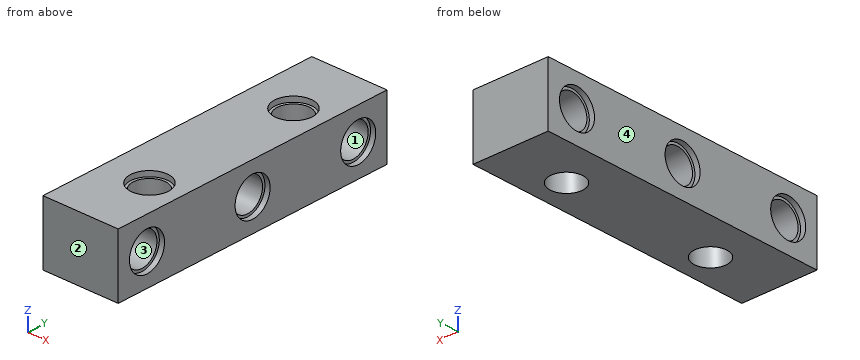
from build123d import *

# Parameters (mm, degrees)
ESQUISSE1_W                  = 12
ESQUISSE1_H                  = 40
BOSS_EXTRU_1_DEPTH           = 12
ESQUISSE3_R                  = 3.15
ENL_V_MAT_EXTRU_1_DEPTH      = 44.451121965
ENL_V_MAT_EXTRU_1_DEPTH_BACK = 44.451121965
ESQUISSE4_R                  = 3.15
ENL_V_MAT_EXTRU_2_DEPTH      = 44.451121965
ENL_V_MAT_EXTRU_2_DEPTH_BACK = 44.451121965
ESQUISSE5_R                  = 3.65
ENL_V_MAT_EXTRU_3_DEPTH      = 1
ESQUISSE6_R                  = 3.65
ENL_V_MAT_EXTRU_4_DEPTH      = 1
ESQUISSE7_W                  = 12
ESQUISSE7_H                  = 8
BOSS_EXTRU_2_DEPTH           = 12
ESQUISSE8_W                  = 1
ESQUISSE8_H                  = 12
ENL_V_MAT_EXTRU_5_DEPTH      = 59.514955353
ENL_V_MAT_EXTRU_5_DEPTH_BACK = 59.514955353
ESQUISSE9_R                  = 3.15
ENL_V_MAT_EXTRU_6_DEPTH      = 51.68530359
ENL_V_MAT_EXTRU_6_DEPTH_BACK = 51.68530359
ESQUISSE11_W                 = 12
ESQUISSE11_H                 = 56
ESQUISSE11_R                 = 3.15
BOSS_EXTRU_3_DEPTH           = 3.5
ESQUISSE12_R                 = 3.65
ENL_V_MAT_EXTRU_8_DEPTH      = 1
ESQUISSE13_R                 = 3.65
ENL_V_MAT_EXTRU_9_DEPTH      = 1


with BuildPart() as part:
    # Esquisse1 → Boss.-Extru.1 (new body)
    with BuildSketch(Plane.XY):
        with Locations((6, 20)):
            Rectangle(ESQUISSE1_W, ESQUISSE1_H)
    extrude(amount=BOSS_EXTRU_1_DEPTH)

    # Esquisse3 → Enlèv. mat.-Extru.1 (cut, two sides)
    with BuildSketch(Plane.XY.offset(12)) as enl_v_mat_extru_1_sk:
        with Locations((5, 5)):
            Circle(ESQUISSE3_R)
        with Locations((5, 35)):
            Circle(ESQUISSE3_R)
    extrude(amount=ENL_V_MAT_EXTRU_1_DEPTH, mode=Mode.SUBTRACT)
    extrude(enl_v_mat_extru_1_sk.sketch, amount=-ENL_V_MAT_EXTRU_1_DEPTH_BACK, mode=Mode.SUBTRACT)

    # Esquisse4 → Enlèv. mat.-Extru.2 (cut, two sides)
    with BuildSketch(Plane(origin=(12, 0, 0), x_dir=(0, 0, -1), z_dir=(1, 0, 0))) as enl_v_mat_extru_2_sk:
        with Locations((-6, 20)):
            Circle(ESQUISSE4_R)
    extrude(amount=ENL_V_MAT_EXTRU_2_DEPTH, mode=Mode.SUBTRACT)
    extrude(enl_v_mat_extru_2_sk.sketch, amount=-ENL_V_MAT_EXTRU_2_DEPTH_BACK, mode=Mode.SUBTRACT)

    # Esquisse5 → Enlèv. mat.-Extru.3 (cut)
    with BuildSketch(Plane.XY.offset(12)):
        with Locations((5, 35)):
            Circle(ESQUISSE5_R)
        with Locations((5, 5)):
            Circle(ESQUISSE5_R)
    extrude(amount=-ENL_V_MAT_EXTRU_3_DEPTH, mode=Mode.SUBTRACT)

    # Esquisse6 → Enlèv. mat.-Extru.4 (cut)
    with BuildSketch(Plane(origin=(12, 0, 0), x_dir=(0, 0, -1), z_dir=(1, 0, 0))):
        with Locations((-6, 20)):
            Circle(ESQUISSE6_R)
    extrude(amount=-ENL_V_MAT_EXTRU_4_DEPTH, mode=Mode.SUBTRACT)

    # Esquisse7 → Boss.-Extru.2 (add)
    with BuildSketch(Plane(origin=(12, 0, 0), x_dir=(0, 0, -1), z_dir=(1, 0, 0))):
        with Locations((-6, -4)):
            Rectangle(ESQUISSE7_W, ESQUISSE7_H)
        with Locations((-6, 44)):
            Rectangle(ESQUISSE7_W, ESQUISSE7_H)
    extrude(amount=-BOSS_EXTRU_2_DEPTH)

    # Esquisse8 → Enlèv. mat.-Extru.5 (cut, two sides)
    with BuildSketch(Plane.XZ.offset(8)) as enl_v_mat_extru_5_sk:
        with Locations((11.5, 6)):
            Rectangle(ESQUISSE8_W, ESQUISSE8_H)
    extrude(amount=ENL_V_MAT_EXTRU_5_DEPTH, mode=Mode.SUBTRACT)
    extrude(enl_v_mat_extru_5_sk.sketch, amount=-ENL_V_MAT_EXTRU_5_DEPTH_BACK, mode=Mode.SUBTRACT)

    # Esquisse9 → Enlèv. mat.-Extru.6 (cut, two sides)
    with BuildSketch(Plane(origin=(11, 0, 0), x_dir=(0, 0, -1), z_dir=(1, 0, 0))) as enl_v_mat_extru_6_sk:
        with Locations((-6, 42)):
            Circle(ESQUISSE9_R)
        with Locations((-6, -2)):
            Circle(ESQUISSE9_R)
    extrude(amount=ENL_V_MAT_EXTRU_6_DEPTH, mode=Mode.SUBTRACT)
    extrude(enl_v_mat_extru_6_sk.sketch, amount=-ENL_V_MAT_EXTRU_6_DEPTH_BACK, mode=Mode.SUBTRACT)

    # Esquisse11 → Boss.-Extru.3 (add)
    with BuildSketch(Plane.ZY):
        with Locations((6, 20)):
            Rectangle(ESQUISSE11_W, ESQUISSE11_H)
        with Locations(Location((6, -2, 0), (0, 0, 180))):
            Circle(ESQUISSE11_R, mode=Mode.SUBTRACT)
        with Locations(Location((6, 20, 0), (0, 0, 180))):
            Circle(ESQUISSE11_R, mode=Mode.SUBTRACT)
        with Locations(Location((6, 42, 0), (0, 0, 180))):
            Circle(ESQUISSE11_R, mode=Mode.SUBTRACT)
    extrude(amount=BOSS_EXTRU_3_DEPTH)

    # Esquisse12 → Enlèv. mat.-Extru.8 (cut)
    with BuildSketch(Plane.ZY.offset(3.5)):
        with Locations((6, 42)):
            Circle(ESQUISSE12_R)
        with Locations((6, 20)):
            Circle(ESQUISSE12_R)
        with Locations((6, -2)):
            Circle(ESQUISSE12_R)
    extrude(amount=-ENL_V_MAT_EXTRU_8_DEPTH, mode=Mode.SUBTRACT)

    # Esquisse13 → Enlèv. mat.-Extru.9 (cut)
    with BuildSketch(Plane(origin=(11, 0, 0), x_dir=(0, 0, -1), z_dir=(1, 0, 0))):
        with Locations(Location((-6, -2, 0), (0, 0, 180))):
            Circle(ESQUISSE13_R)
        with Locations(Location((-6, 20, 0), (0, 0, 180))):
            Circle(ESQUISSE13_R)
        with Locations(Location((-6, 42, 0), (0, 0, 180))):
            Circle(ESQUISSE13_R)
    extrude(amount=-ENL_V_MAT_EXTRU_9_DEPTH, mode=Mode.SUBTRACT)


solid = part.part
The listing builds one solid part. Answer for the finished solid, in the listing's coordinates (mm). Face numbers are marked on the shaded views. Coordinates: 2 decimals unless noted, no trailing zeros. Loops run counter-clockwise (first coordinate to the right, second up) from the corner with the lowest first, then second, coordinate; pieces in that order, holes last. Notation, with made-up numbers: (78, -27) -> (87, -27) arc R27 ccw to (87, -9) -> close; hole circle Ø7 at (-34, 34). An arc over 180 degrees is marked (long way). Write item = value, one per line. Start each with the question number.
1) Given pin 1 Ø2 at (y, z) = (19.5, 4) entering from -X; pin 2 Ø2 at (y, z) = (43.5, 8) entering from -X, each flat-ended and moving along its own axis, determine where each tip first touches the part or whether it passes through.
2) A cutting plane is placed at D-D (z = 6). Count the separate pieces of the cut face and the enclosed holes in it, then the cut area to 3 significant figures.
3) A cutting plane is placed at C-C (x = -0.5). Give the vertices of the cut face in (y, z).
4) Straight lines are drawn through the part: line 1 (Y direction, x = 5, z = 11.35); line 2 (Y direction, x = -2.65, z = 6); line 3 (Y direction, x = 4.75, z = 6.75). For each, find the intervals that lie inside material, in ascending order. Write a range as from..to.
5) A cutting plane is placed at B-B (x = 5). Give the vertices of the cut face in (y, z), then the cut area to 3 significant figures.
6) A cutting plane is placed at A-A (y = 35). Give the vertices of the cut face in (x, z), then the cut area to 3 significant figures.
7) The mould has two halves that part along Y. Classify the marked faces 1, 2, 3 and 4: released by +Y, released by -Y, zero draft, split by the parting line, or undercut.
Responses:
q1.pin_1 = through
q1.pin_2 = -2.5
q2.separate_pieces = 4
q2.enclosed_holes = 2
q2.area = 470 mm²
q3.outline = (-8, 0) -> (48, 0) -> (48, 12) -> (-8, 12) -> close; hole circle Ø6.3 at (-2, 6); hole circle Ø6.3 at (20, 6); hole circle Ø6.3 at (42, 6)
q4.line_1 = -8..1.35, 8.65..31.35, 38.65..48
q4.line_2 = -8..-5.65, 1.65..16.35, 23.65..38.35, 45.65..48
q4.line_3 = -8..-5.06, 1.06..1.86, 8.14..16.94, 23.06..31.86, 38.14..38.94, 45.06..48
q5.outline = (-8, 0) -> (1.85, 0) -> (1.85, 11) -> (1.35, 11) -> (1.35, 12) -> (-8, 12) -> close; (8.15, 0) -> (31.85, 0) -> (31.85, 11) -> (31.35, 11) -> (31.35, 12) -> (8.65, 12) -> (8.65, 11) -> (8.15, 11) -> close; (38.15, 0) -> (48, 0) -> (48, 12) -> (38.65, 12) -> (38.65, 11) -> (38.15, 11) -> close; hole circle Ø6.3 at (-2, 6); hole circle Ø6.3 at (20, 6); hole circle Ø6.3 at (42, 6)
q5.area = 425 mm²
q6.outline = (-3.5, 0) -> (1.85, 0) -> (1.85, 11) -> (1.35, 11) -> (1.35, 12) -> (-3.5, 12) -> close; (8.15, 0) -> (11, 0) -> (11, 12) -> (8.65, 12) -> (8.65, 11) -> (8.15, 11) -> close
q6.area = 97.4 mm²
q7.face_1 = undercut
q7.face_2 = released by -Y
q7.face_3 = undercut
q7.face_4 = zero draft
